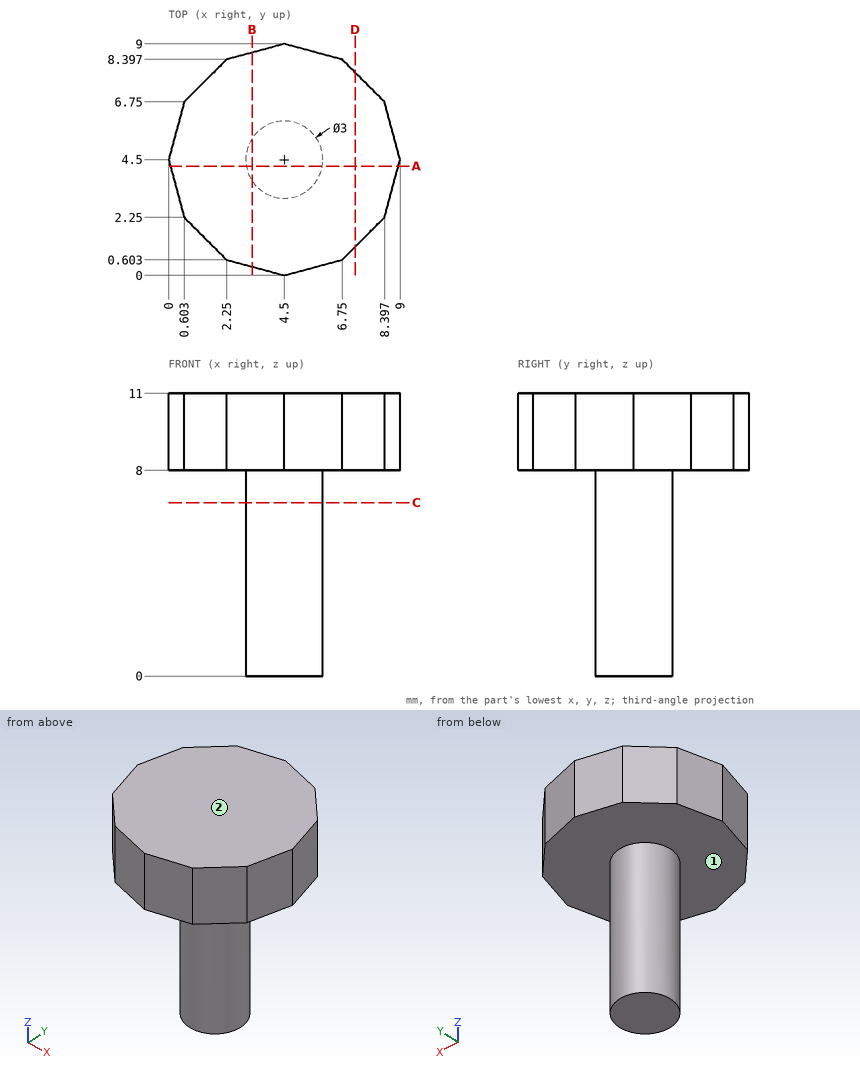
Study the drawing (mm; zero at the part's minimum x, y, z) and answer. A direction names the side the tool comes from. Coordinates: 2 decimals unless noted, no trailing zeros. Write each loop counter-clockwise with the first axis right and the second up, starting at its lowest first coordinate (ties: lowest second). Pieces come first, ordered by that corner, then holes. Notation, with made-up numbers: (-10, 30) - (39, 30) arc R18 cw to (39, 57) - close; hole circle Ø9 at (-35.5, 47.25). An arc over 180 degrees is marked (long way). Answer as a JSON object with one key per item and string values. Group by question number.
1. A cutting plane is placed at C-C (z = 6.75). Determine the outline of the cut face in (x, y), plus the area to 3 significant figures.
2. A cutting plane is placed at D-D (x = 7.25). Determine the outline of the cut face in (y, z).
3. Each of these flat-tipped pins is pushed along its axis until it touches: P1, Ø5, axis at y = 1.5, z = 5, coming from the +X side; P2, Ø1, axis at x = 1.5, y = 1, coming from the -Z side. Where does it stop, or does it pass through?
4. Consider L1, parallel to Z at x = 1.75, y = 6.25; L2, parallel to X at y = 3.25, z = 3.25; L3, parallel to Y at x = 4, z = 8.25. Determine where each line is inside the solid, lowest interval first. Write a range as [from, to].
5. Which of the six approach directions +Z, -Z, +X, -X, +Y, -Y give full straight-line access (tool end or side, diameter ignored) to the marked faces 1 and 2?
6. A cutting plane is placed at B-B (x = 3.25). Determine the outline of the cut face in (y, z) (3 decimals).
7. A cutting plane is placed at A-A (y = 4.25). Determine the outline of the cut face in (x, z).
Worked out:
{
 "1": {"outline": "circle Ø3 at (4.5, 4.5)", "area": "7.07 mm²"},
 "2": {"outline": "(1.1, 8) - (7.9, 8) - (7.9, 11) - (1.1, 11) - close"},
 "3": {"P1": "stops at x = 5.91", "P2": "stops at z = 8"},
 "4": {"L1": "z = [8, 11]", "L2": "x = [3.67, 5.33]", "L3": "y = [0.13, 8.87]"},
 "5": {"face 1": "-Z", "face 2": "+Z, +X, -X, +Y, -Y"},
 "6": {"outline": "(0.335, 8) - (3.671, 8) - (3.671, 0) - (5.329, 0) - (5.329, 8) - (8.665, 8) - (8.665, 11) - (0.335, 11) - close"},
 "7": {"outline": "(0.07, 8) - (3.02, 8) - (3.02, 0) - (5.98, 0) - (5.98, 8) - (8.93, 8) - (8.93, 11) - (0.07, 11) - close"}
}
